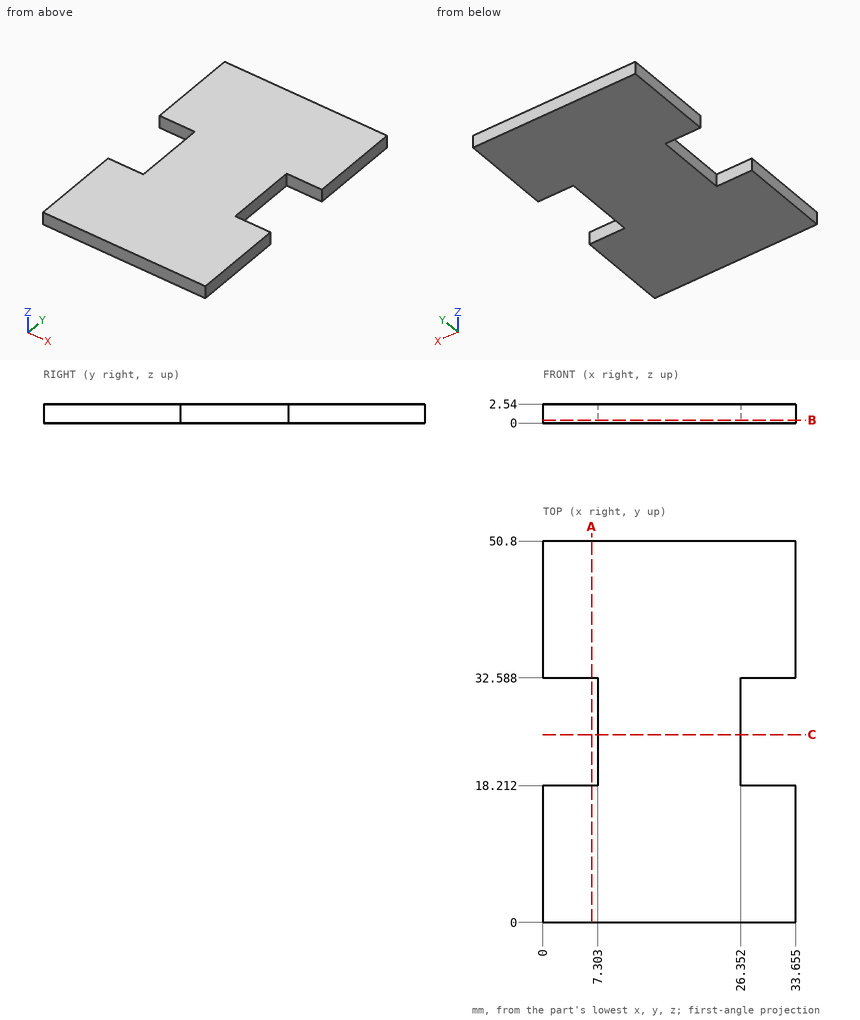
Drawing for the job (mm, zero at the part's lowest x, y, z). Round coordinates to 2 decimals unless told otherwise and drop trailing zeros. Order: outer loops, then holes, each group sorted by start corner. A loop starts at its lowest first (then second) coordinate and runs counter-clockwise, first axis right, second up. Notation, with made-up numbers: (-21, 72) -> (-3, 72) arc R12 ccw to (-3, 80) -> close; hole circle Ø3 at (38.5, 51). An arc over 180 degrees is marked (long way). Write item = value, one per line. Start each with the question number.
(1) Probe line 1 (Y direction, x = 5.5, z = 2.4); line 2 (X direction, y = 22, z = 0.65). List the from-to ranges inside material, lowest first. Write a range as [from, to].
(2) Cut at B-B, the plane z = 0.4. List the corners of the cut face in (x, y) (1 decimal), then the cut area to 3 significant figures.
(3) Cut at A-A, the plane x = 6.5. List the corners of the cut face in (y, z).
(4) Cut at C-C, the plane y = 25. List the corners of the cut face in (x, z).
(5) Pin check, flat tips, straight feed: P1, Ø0.8, axis at y = 24, z = 1, coming from the -X side; P2, Ø1.3, axis at y = 28.5, z = 1.5, coming from the +X side. Stop position of each tip, or through.
Model answer:
q1.line_1 = [0, 18.21], [32.59, 50.8]
q1.line_2 = [7.3, 26.35]
q2.outline = (0, 0) -> (33.7, 0) -> (33.7, 18.2) -> (26.4, 18.2) -> (26.4, 32.6) -> (33.7, 32.6) -> (33.7, 50.8) -> (0, 50.8) -> (0, 32.6) -> (7.3, 32.6) -> (7.3, 18.2) -> (0, 18.2) -> close
q2.area = 1,500 mm2
q3.outline = (0, 0) -> (18.21, 0) -> (18.21, 2.54) -> (0, 2.54) -> close; (32.59, 0) -> (50.8, 0) -> (50.8, 2.54) -> (32.59, 2.54) -> close
q4.outline = (7.3, 0) -> (26.35, 0) -> (26.35, 2.54) -> (7.3, 2.54) -> close
q5.P1 = 7.3
q5.P2 = 26.35
